The listing builds one solid part. Answer for the finished solid, in the listing's coordinates (mm). A direction names the side the tool comes from. Round coordinates to 2 decimals unless told otherwise and drop trailing zeros. Order: outer loops, then holes, each group sorted by start corner. A loop starts at its lowest first (then second) coordinate and runs counter-clockwise, first axis right, second up. Notation, with made-up numbers: M -8.5,0 L 33.5,0 A16 cw 33.5,10 Z; hole C 6.25,-22 d7. An arc over 180 degrees is marked long. Put each result on its own line as item: value. Start each with the question number.
1. The mould has two halves that part along X. Classify faces 1 (the face through (1, 0, 3)), 2 (the face through (10.913, 3.869, -0.042)): +X half, -X half, draft (parallel to the pull), parting line (faces both ways), or undercut.
2. Which of the six approach directions +Z, -Z, +X, -X, +Y, -Y give full straight-line access (tool end or side, diameter ignored) to faces 3 (the face through (-1, 3.5, 0)), 4 (the face through (1, 0, -3))?
3. Consider line 1 (X direction, y = 0.25, z = -0.4); line 2 (X direction, y = -1.25, z = -1); line 3 (Y direction, x = 19.5, z = 0.9). Determine where each line is inside the solid, lowest interval first.
4. The part is cut by section D-D (y = -6). Give the vertices of the cut face in (x, z).
5. The part is cut by section C-C (x = 6.5). Give the vertices of the cut face in (y, z), then the cut area to 3 significant figures.
6. The part is cut by section B-B (z = -0.6). Give the vertices of the cut face in (x, y).
7. The part is cut by section A-A (x = 19). Give the vertices of the cut face in (y, z), then the cut area to 3 significant figures.
8. Each of these flat-tipped pins is pushed along its axis until it touches: pin 1 Ø1.5 at (y, z) = (-1, 1) entering from -X; pin 2 Ø0.9 at (x, z) = (-2, 1) entering from -Y; pin 3 Ø1 at (x, z) = (8, -0.5) entering from +Y. Where does it stop, or does it pass through?
from build123d import *

# Parameters (mm, degrees)
BOSS_EXTRUDE1_DEPTH = 3
FILLET1_R           = 5


with BuildPart() as part:
    # Sketch3 → Boss-Extrude1 (new, symmetric)
    with BuildSketch(Plane.XY):
        with BuildLine():
            Line((11.437822174, 3.5), (-13.929285786, 3.5))
            ThreePointArc((-13.929285786, 3.5), (-12.871092404, 1.890294809), (-12.5, 0))
            ThreePointArc((-12.5, 0), (-12.871092404, -1.890294809), (-13.929285786, -3.5))
            Line((-13.929285786, -3.5), (11.437822174, -3.5))
            ThreePointArc((11.437822174, -3.5), (10.5, 0), (11.437822174, 3.5))
        make_face()
        with BuildLine():
            Line((-17.5, 3), (-17.5, 3.5))
            Line((-17.5, 3.5), (-13.929285786, 3.5))
            ThreePointArc((-13.929285786, 3.5), (-22.5, 0), (-13.929285786, -3.5))
            Line((-13.929285786, -3.5), (-17.5, -3.5))
            Line((-17.5, -3.5), (-17.5, -3))
            ThreePointArc((-17.5, -3), (-20.5, 0), (-17.5, 3))
        make_face()
        with BuildLine():
            Line((-13.929285786, 3.5), (-17.5, 3.5))
            Line((-17.5, 3.5), (-17.5, 3))
            ThreePointArc((-17.5, 3), (-15.378679656, 2.121320344), (-14.5, 0))
            ThreePointArc((-14.5, 0), (-15.378679656, -2.121320344), (-17.5, -3))
            Line((-17.5, -3), (-17.5, -3.5))
            Line((-17.5, -3.5), (-13.929285786, -3.5))
            ThreePointArc((-13.929285786, -3.5), (-12.871092404, -1.890294809), (-12.5, 0))
            ThreePointArc((-12.5, 0), (-12.871092404, 1.890294809), (-13.929285786, 3.5))
        make_face()
        with BuildLine():
            ThreePointArc((24.5, 0), (19.311733316, 6.761480784), (11.437822174, 3.5))
            Line((11.437822174, 3.5), (15.563508327, 3.5))
            ThreePointArc((15.563508327, 3.5), (19.531506006, 3.445719569), (21.5, 0))
            ThreePointArc((21.5, 0), (19.531506006, -3.445719569), (15.563508327, -3.5))
            Line((15.563508327, -3.5), (11.437822174, -3.5))
            ThreePointArc((11.437822174, -3.5), (19.311733316, -6.761480784), (24.5, 0))
        make_face()
        with BuildLine():
            Line((15.563508327, 3.5), (11.437822174, 3.5))
            ThreePointArc((11.437822174, 3.5), (10.5, 0), (11.437822174, -3.5))
            Line((11.437822174, -3.5), (15.563508327, -3.5))
            ThreePointArc((15.563508327, -3.5), (13.5, 0), (15.563508327, 3.5))
        make_face()
    extrude(amount=BOSS_EXTRUDE1_DEPTH, both=True)

    # Fillet1
    fillet1_edges = [part.edges().sort_by_distance(p)[0] for p in [
        (-13.929285786, 3.5, 0),
        (11.437822174, 3.5, 0),
        (11.437822174, -3.5, 0),
        (-13.929285786, -3.5, 0),
    ]]
    fillet(fillet1_edges, radius=FILLET1_R)


solid = part.part
Resolved:
1. face 1: draft
1. face 2: undercut
2. face 3: +Z, -Z, +Y
2. face 4: -Z, +X, -X, +Y, -Y
3. line 1: -22.49 to -20.49, -14.51 to 13.51, 21.49 to 24.5
3. line 2: -22.34 to -20.23, -14.77 to 13.7, 21.3 to 24.39
3. line 3: -6.71 to -3.46, 3.46 to 6.71
4. outline: M 13.89,-3 L 21.11,-3 L 21.11,3 L 13.89,3 Z
5. outline: M -3.5,-3 L 3.5,-3 L 3.5,3 L -3.5,3 Z
5. area: 42.0 mm2
6. outline: M -14.87,-4.25 A5 cw -12.23,-3.5 L 9.03,-3.5 A5 cw 12.56,-4.96 A7 ccw long 12.56,4.96 A5 cw 9.03,3.5 L -12.23,3.5 A5 cw -14.87,4.25 A5 ccw long Z; hole C -17.5,0 d6; hole C 17.5,0 d8
7. outline: M -6.84,-3 L -3.71,-3 L -3.71,3 L -6.84,3 Z; M 3.71,-3 L 6.84,-3 L 6.84,3 L 3.71,3 Z
7. area: 37.6 mm2
8. pin 1: x = -22.49
8. pin 2: y = -3.5
8. pin 3: y = 3.5
